Geometry: final body of the model. Coordinates: model frame, mm. Round coordinates to 2 decimals unless told otherwise and drop trailing zeros. Loops run counter-clockwise (first coordinate to the right, second up) from the corner with the lowest first, then second, coordinate; pieces in that order, holes last. Notation, with made-up numbers: (62.5, 57) - (114.5, 57) arc R16 ccw to (114.5, 81) - close; hole circle Ø8 at (12.25, -24). An arc over 180 degrees is marked (long way). Use CSV: the item, a comma, the result in double quotes.
from build123d import *

# Parameters (mm, degrees)
SKETCH_1_W          = 46
SKETCH_1_H          = 46
SKETCH_1_R          = 1.6
SKETCH_1_R_2        = 1.15
EXTRUDE_1_DEPTH     = 3
FILLET_1_R          = 3
SKETCH_2_W          = 22
SKETCH_2_H          = 20
CUT_EXTRUDE_1_DEPTH = 3
FILLET_2_R          = 3


with BuildPart() as part:
    # 草图1 → 凸台-拉伸1 (new body)
    with BuildSketch(Plane.XY):
        Rectangle(SKETCH_1_W, SKETCH_1_H)
        with Locations((-20, 20)):
            Circle(SKETCH_1_R, mode=Mode.SUBTRACT)
        with Locations((20, 20)):
            Circle(SKETCH_1_R, mode=Mode.SUBTRACT)
        with Locations((20, -20)):
            Circle(SKETCH_1_R, mode=Mode.SUBTRACT)
        with Locations((-20, -20)):
            Circle(SKETCH_1_R, mode=Mode.SUBTRACT)
        with Locations((-14.7, 8.7)):
            Circle(SKETCH_1_R_2, mode=Mode.SUBTRACT)
        with Locations((14.7, 8.7)):
            Circle(SKETCH_1_R_2, mode=Mode.SUBTRACT)
        with Locations((14.7, -8.7)):
            Circle(SKETCH_1_R_2, mode=Mode.SUBTRACT)
        with Locations((-14.7, -8.7)):
            Circle(SKETCH_1_R_2, mode=Mode.SUBTRACT)
    extrude(amount=EXTRUDE_1_DEPTH)

    # 圆角1
    fillet_1_edges = [part.edges().sort_by_distance(p)[0] for p in [
        (-23, 23, 1.5),
        (23, 23, 1.5),
        (23, -23, 1.5),
        (-23, -23, 1.5),
    ]]
    fillet(fillet_1_edges, radius=FILLET_1_R)

    # 草图2 → 切除-拉伸1 (cut)
    with BuildSketch(Plane.XY.offset(3)):
        Rectangle(SKETCH_2_W, SKETCH_2_H)
    extrude(amount=-CUT_EXTRUDE_1_DEPTH, mode=Mode.SUBTRACT)

    # 圆角2
    fillet_2_edges = [part.edges().sort_by_distance(p)[0] for p in [
        (-11, -10, 1.5),
        (-11, 10, 1.5),
        (11, 10, 1.5),
        (11, -10, 1.5),
    ]]
    fillet(fillet_2_edges, radius=FILLET_2_R)


solid = part.part
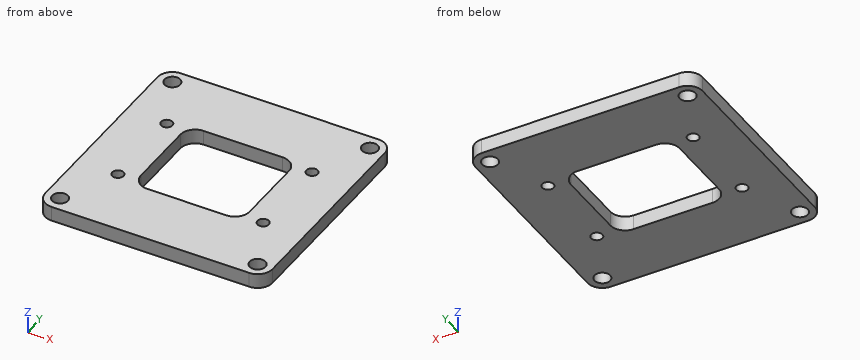
Item 1: Section C-C on z = 1.9. Give the number of separate pieces and of enclosed holes in the cut face, plus the area to 3 significant figures.
Final values:
separate pieces,"1"
enclosed holes,"9"
area,"1,630 mm²"
Item 2: Section D-D on x = 14.7. Return the cut outline in (y, z).
Final values:
outline,"(-23, 0) - (-9.85, 0) - (-9.85, 3) - (-23, 3) - close; (-7.55, 0) - (7.55, 0) - (7.55, 3) - (-7.55, 3) - close; (9.85, 0) - (23, 0) - (23, 3) - (9.85, 3) - close"
Item 3: Material intervals for line 1 (Y direction, x = 14.7, z = 2.25); line 2 (Y direction, x = 20, z = 1.85); line 3 (Y direction, x = -1, z = 2.05), sorted ascending.
Final values:
line 1,"y = -23 to -9.85, -7.55 to 7.55, 9.85 to 23"
line 2,"y = -23 to -21.6, -18.4 to 18.4, 21.6 to 23"
line 3,"y = -23 to -10, 10 to 23"
Item 4: Section B-B on x = -3. Return the cut outline in (y, z).
Final values:
outline,"(-23, 0) - (-10, 0) - (-10, 3) - (-23, 3) - close; (10, 0) - (23, 0) - (23, 3) - (10, 3) - close"
Item 5: Section A-A on y = 1. Return the cut outline in (x, z).
Final values:
outline,"(-23, 0) - (-11, 0) - (-11, 3) - (-23, 3) - close; (11, 0) - (23, 0) - (23, 3) - (11, 3) - close"
